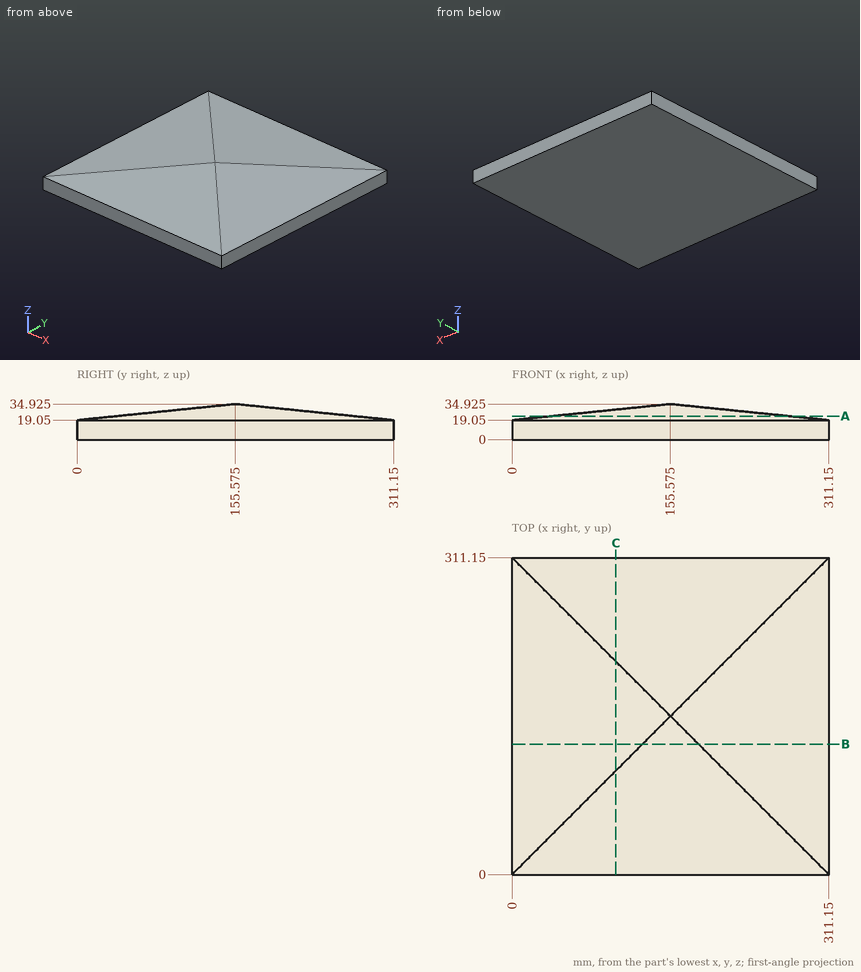
Check sheet for the drawn part. Datum: minimum x, y, z corner. Units: mm. Give positions to 0.01 mm unless a question says otherwise; leave off trailing zeros. Write each loop counter-clockwise with the first axis right and the second up, starting at its lowest first coordinate (ties: lowest second). Pieces come first, ordered by that corner, then holes.
(1) Gauge pin test, flat ends, axial feed: pin 1 (2 mm diameter, centred on x = 148, y = 176.5, fed in from +Z); pin 2 (2 mm diameter, centred on x = 190, y = 59, fed in from +Z). Record the tip position at first contact, or that the pin passes through.
(2) Cross-section at A-A (z = 23). Enter the section's corners in (x, y).
(3) Cross-section at C-C (x = 102). Enter the section's corners in (y, z), plus the area to 3 significant figures.
(4) Material ranges on line 1 (Z direction, x = 34, y = 157); line 2 (Z direction, x = 225.5, y = 91.5), recorded low to high.
(5) Cross-section at B-B (y = 128). Enter the section's corners in (x, z), plus the area to 3 significant figures.
Worked out:
1. pin 1: stops at z = 32.89
1. pin 2: stops at z = 25.17
2. outline: (38.71, 38.71) - (272.44, 38.71) - (272.44, 272.44) - (38.71, 272.44) - close
3. outline: (0, 0) - (311.15, 0) - (311.15, 19.05) - (209.15, 29.46) - (102, 29.46) - (0, 19.05) - close
3. area: 8,100 mm2
4. line 1: z = 0 to 22.52
4. line 2: z = 0 to 27.79
5. outline: (0, 0) - (311.15, 0) - (311.15, 19.05) - (183.15, 32.11) - (128, 32.11) - (0, 19.05) - close
5. area: 8,320 mm2
